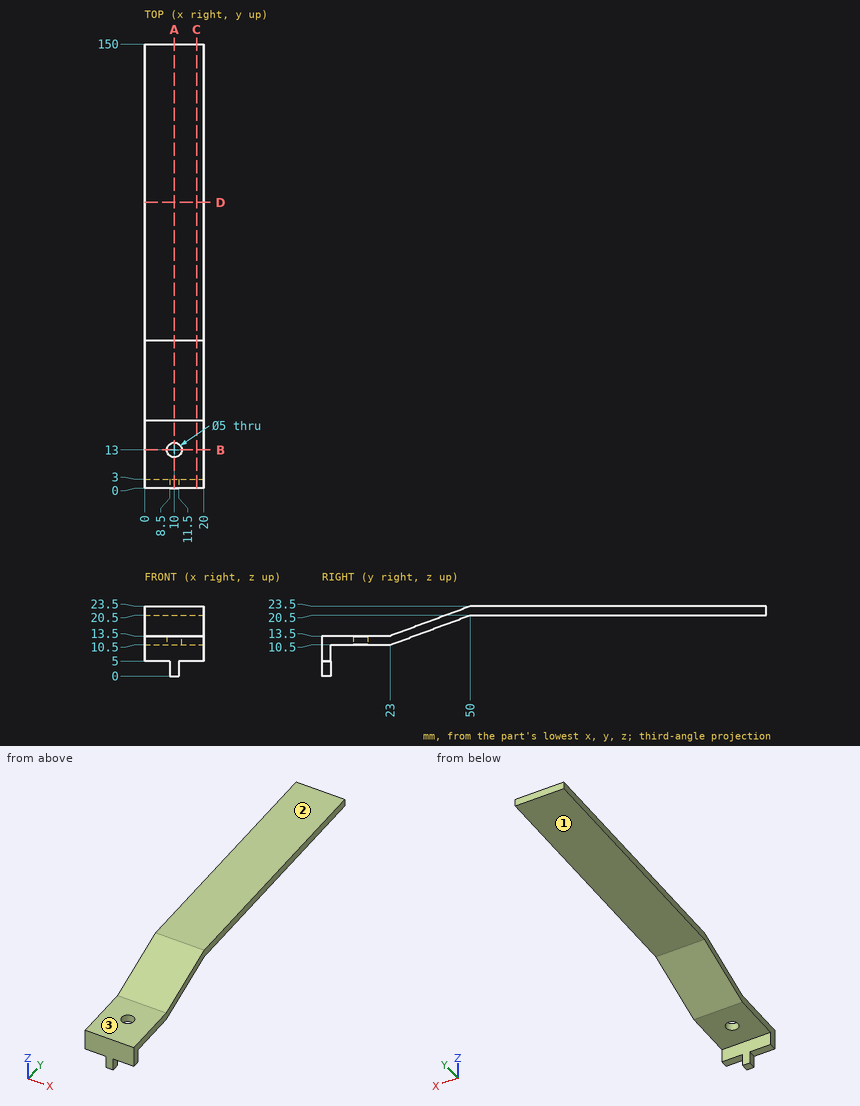
The drawing under review shows one solid part. Ordinate dimensions are in mm from its lowest x, y, z. A direction names the side the tool comes from. Give positions to 0.01 mm unless a question says otherwise; leave off trailing zeros. Loops run counter-clockwise (first coordinate to the right, second up) from the corner with the lowest first, then second, coordinate; pieces in that order, holes last. Notation, with made-up numbers: M 15,-17 L 24,-17 A20 cw 24,-8 Z; hole C -35.75,32 d5. An arc over 180 degrees is marked long. One line per item, written item: value. Start each with the question number.
Q1. For L1, parallel to X at y = 13, z = 11.9; L2, parallel to Z at x = 11, y = 135.5; L3, parallel to Z at x = 7, y = 20.5, list the stretches that pass through material, from the lowest coordinate up.
Q2. Add section D-D (y = 96.5). Give the boundary of the cut face in (x, z), and give its area (3 significant figures).
Q3. Add section B-B (y = 13). Give the boundary of the cut face in (x, z), and give its area (3 significant figures).
Q4. Clearance check with flat-ended pins moving along their axes: pin 1 Ø4 at (x, y) = (11.5, 115.5) entering from -Z; pin 2 Ø0.9 at (y, z) = (1, 3.5) entering from +X; pin 3 Ø10 at (x, y) = (13, 13.5) entering from -Z; pin 4 Ø6 at (x, z) = (4, 13) entering from -Y. State where each tip first meets the part, or that it passes through.
Q5. Add section A-A (x = 10). Give the boundary of the cut face in (y, z), and give its area (4 significant figures).
Q6. Machinability: for the marked faces 1, 2 and 3, which of the approach directions +Z, -Z, +X, -X, +Y, -Y give a long, thin tool a straight path to every point of the face, cutting with its end or side? Answer none if there is none.
Q7. Add section C-C (x = 17.5). Give the boundary of the cut face in (y, z), and give its area (4 significant figures).
Reply:
1. L1: 0 to 7.5, 12.5 to 20
1. L2: 20.5 to 23.5
1. L3: 10.5 to 13.5
2. outline: M 0,20.5 L 20,20.5 L 20,23.5 L 0,23.5 Z
2. area: 60.0 mm²
3. outline: M 0,10.5 L 7.5,10.5 L 7.5,13.5 L 0,13.5 Z; M 12.5,10.5 L 20,10.5 L 20,13.5 L 12.5,13.5 Z
3. area: 45.0 mm²
4. pin 1: z = 20.5
4. pin 2: x = 11.5
4. pin 3: z = 10.5
4. pin 4: y = 0
5. outline: M 0,0 L 3,0 L 3,10.5 L 10.5,10.5 L 10.5,13.5 L 0,13.5 Z; M 15.5,10.5 L 23,10.5 L 50,20.5 L 150,20.5 L 150,23.5 L 50,23.5 L 23,13.5 L 15.5,13.5 Z
5. area: 466.5 mm²
6. face 1: -Z, +X, -X, +Y
6. face 2: +Z, +X, -X, +Y, -Y
6. face 3: +Z, +X, -X, -Y
7. outline: M 0,5 L 3,5 L 3,10.5 L 23,10.5 L 50,20.5 L 150,20.5 L 150,23.5 L 50,23.5 L 23,13.5 L 0,13.5 Z
7. area: 466.5 mm²
